The listing builds one solid part. Answer for the finished solid, in the listing's coordinates (mm). Give positions to 0.01 mm unless a question says otherwise; leave off trailing zeros. Order: outer loops, then holes, each group sorted by start corner. A loop starts at its lowest first (then second) coordinate and runs counter-clockwise, first axis right, second up. Notation, with made-up numbers: (-20, 23) - (24, 23) arc R30 ccw to (24, 57) - close; hole circle Ø5 at (58.25, 60). An arc over 180 degrees is marked (long way). Use CSV: the item, a comma, the result in double quotes.
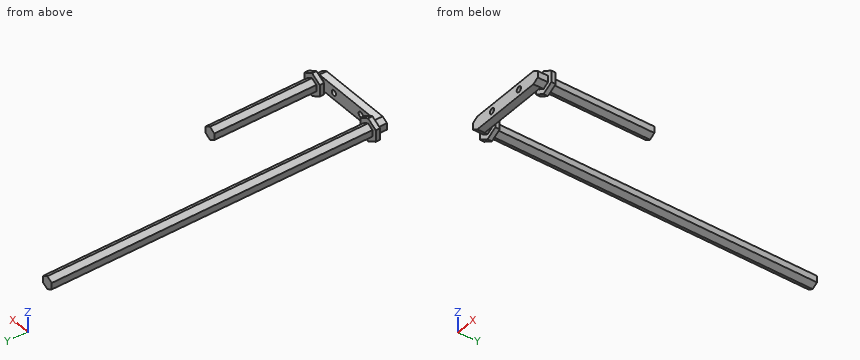
```python
from build123d import *

# Parameters (mm, degrees)
SKETCH1_W           = 50
SKETCH1_H           = 9
SKETCH1_R           = 1.9
BOSS_EXTRUDE1_DEPTH = 5
BOSS_EXTRUDE2_DEPTH = 80
BOSS_EXTRUDE3_DEPTH = 150
BOSS_EXTRUDE4_DEPTH = 3


with BuildPart() as part:
    # Sketch1 → Boss-Extrude1 (new body)
    with BuildSketch(Plane(origin=(0, 0, 0), x_dir=(1, 0, 0), z_dir=(0, 1, 0))):
        with Locations((12, 0)):
            Rectangle(SKETCH1_W, SKETCH1_H)
        with Locations(Location((24, 0, 0), (0, 0, 270))):
            Circle(SKETCH1_R, mode=Mode.SUBTRACT)
        with Locations(Location((0, 0, 0), (0, 0, 270))):
            Circle(SKETCH1_R, mode=Mode.SUBTRACT)
    extrude(amount=BOSS_EXTRUDE1_DEPTH)

    # Sketch3 → Boss-Extrude2 (add)
    with BuildSketch(Plane.XZ):
        Polygon((-13, 4.5), (-16.897114317, 2.25), (-16.897114317, -2.25), (-13, -4.5), (-9.102885683, -2.25), (-9.102885683, 2.25), align=None)
        Polygon((33.102885683, 2.25), (37, 4.5), (40.897114317, 2.25), (40.897114317, -2.25), (37, -4.5), (33.102885683, -2.25), align=None)
    extrude(amount=-BOSS_EXTRUDE2_DEPTH)

    # Sketch4 → Boss-Extrude3 (add)
    with BuildSketch(Plane(origin=(0, 80, 0), x_dir=(1, 0, 0), z_dir=(0, 1, 0))):
        Polygon((-13, -4.5), (-9.102885683, -2.25), (-9.102885683, 2.25), (-13, 4.5), (-16.897114317, 2.25), (-16.897114317, -2.25), align=None)
    extrude(amount=BOSS_EXTRUDE3_DEPTH)

    # Sketch5 → Boss-Extrude4 (add)
    # profile 1 of 2: a face of its own
    with BuildSketch(Plane(origin=(0, 7, 0), x_dir=(-1, 0, 0), z_dir=(0, -1, 0))):
        Polygon((19.897114317, 3.982050808), (19.897114317, -3.982050808), (13, -7.964101615), (6.102885683, -3.982050808), (6.102885683, 3.982050808), (13, 7.964101615), align=None)
        Polygon((16.897114317, -2.25), (13, -4.5), (9.102885683, -2.25), (9.102885683, 2.25), (13, 4.5), (16.897114317, 2.25), align=None, mode=Mode.SUBTRACT)
    # profile 2 of 2: a face of its own
    with BuildSketch(Plane(origin=(0, 7, 0), x_dir=(-1, 0, 0), z_dir=(0, -1, 0))):
        Polygon((-43.897114317, -3.982050808), (-43.897114317, 3.982050808), (-37, 7.964101615), (-30.102885683, 3.982050808), (-30.102885683, -3.982050808), (-37, -7.964101615), align=None)
        Polygon((-33.102885683, 2.25), (-33.102885683, -2.25), (-37, -4.5), (-40.897114317, -2.25), (-40.897114317, 2.25), (-37, 4.5), align=None, mode=Mode.SUBTRACT)
    extrude(amount=-BOSS_EXTRUDE4_DEPTH)


solid = part.part
```
Item 1: The part is cut by section A-A (y = 51). Give the vertices of the cut face in (x, z).
Taken from the geometry:
outline,"(-16.9, -2.25) - (-13, -4.5) - (-9.1, -2.25) - (-9.1, 2.25) - (-13, 4.5) - (-16.9, 2.25) - close; (33.1, -2.25) - (37, -4.5) - (40.9, -2.25) - (40.9, 2.25) - (37, 4.5) - (33.1, 2.25) - close"
Item 2: The part is cut by section C-C (x = 18.5). Give the vertices of the cut face in (y, z).
Taken from the geometry:
outline,"(0, -4.5) - (5, -4.5) - (5, 4.5) - (0, 4.5) - close"
Item 3: The part is cut by section B-B (y = 179.5). Give the vertices of the cut face in (x, z), and give its area (3 significant figures).
Taken from the geometry:
outline,"(-16.9, -2.25) - (-13, -4.5) - (-9.1, -2.25) - (-9.1, 2.25) - (-13, 4.5) - (-16.9, 2.25) - close"
area,"52.6 mm^2"
Item 4: Each of these flat-tipped pins is pushed along its axis until it touches: pin 1 (1.5 mm diameter, centred on x = -8, y = 159, fed in from +Z); pin 2 (3.5 mm diameter, centred on y = 124.5, z = 1, fed in from -X); pin 3 (5 mm diameter, centred on y = 40, z = 0, fed in from +X); pin 4 (2 mm diameter, centred on y = 6.5, z = -0.5, fed in from -X). Where does it stop, or does it pass through?
Taken from the geometry:
pin 1,"through"
pin 2,"x = -16.9"
pin 3,"x = 40.9"
pin 4,"x = -19.9"
Item 5: Find the intervals of material crossed by line 1 along X through (y, z) = (2.95, 0); line 2 along Y through (x, z) = (-7, -2.5); line 3 along X through (y, z) = (24, -1.5), in increasing order.
Taken from the geometry:
line 1,"-16.9 to -1.9, 1.9 to 22.1, 25.9 to 40.9"
line 2,"0 to 5, 7 to 10"
line 3,"-16.9 to -9.1, 33.1 to 40.9"
